Could you check a few things on this model? Use its own coordinates, in mm. A direction names the side the tool comes from. Give positions to 0.01 mm unless a question says otherwise; leave off trailing zeros. Loops run counter-clockwise (first coordinate to the right, second up) from the corner with the lowest first, then second, coordinate; pieces in that order, holes last.
1. Imagine slicing it at A-A (y = 17.5). List the corners of the cut face in (x, z) for me, plus the area to 3 significant figures.
2. Thinking about a two-plate mould opening in Y: for faces 3 (the flat face through (31, -61.113, -3)), 4 (the flat face through (-1, -64.923, -3)), 5 (the flat face through (-68.834, -48, -3)), which applies, +Y half, -Y half, draft (parallel to the pull), parting line (faces both ways), or undercut?
3. For faces 1 (the flat face through (-66, -40, -3)), 2 (the flat face through (-48.11, -15.82, -2.63)), which set-ups out of +Z, -Z, +X, -X, +Y, -Y let a thin tool reach every point of the face, with its end or its side?
4. Imagine slicing it at C-C (x = -34). List the corners of the cut face in (y, z) for me, plus the area to 3 significant figures.
5. I need wall thicknesses on line 1 along X through (y, z) = (1, -2.8); line 2 along X through (y, z) = (-35, -1.9); line 3 along Y through (x, z) = (-37, -2.05). Which ranges of each line are inside material? Lowest first, please.
6. Imagine slicing it at B-B (x = 13). List the corners of the cut face in (y, z) for me, plus the area to 3 significant figures.
7. Imagine slicing it at D-D (z = -2.6). Count the separate pieces of the cut face and the enclosed holes in it, plus the area to 3 significant figures.
8. For P1, Ø1.6, axis at y = 32, z = -3, coming from the +X side; P2, Ø8, axis at x = -30.5, y = -17.5, coming from the -Z side; P3, Ø2.5, axis at y = 5, z = -4, coming from the -X side, each with a flat end and sliding along its axis, tell me the tip position at first contact or that it passes through.
```python
from build123d import *

# Parameters (mm, degrees)
SKETCH1_W                = 127
SKETCH1_H                = 80
TOP_DEPTH                = 5.334
SKETCH2_W                = 127
SKETCH2_H                = 5.334
BOTTOM_DEPTH             = 24.923365698
SKETCH4_W                = 5.334
SKETCH4_H                = 15.24
SKETCH4_H_2              = 12.7
RIGHTTOOTH_DEPTH         = 5.334
SKETCH5_W                = 5.334
SKETCH5_H                = 15.24
SKETCH5_H_2              = 12.7
LEFTTOOTH_DEPTH          = 5.334
SKETCH6_R                = 1.775
PERFBOARDSCREWCUTS_DEPTH = 95.771380308
DESIGN_DEPTH             = 5.334


with BuildPart() as part:
    # Sketch1 → Top (new body)
    with BuildSketch(Plane.XY):
        Rectangle(SKETCH1_W, SKETCH1_H)
    extrude(amount=-TOP_DEPTH)

    # Sketch2 → Bottom (add)
    with BuildSketch(Plane.XZ.offset(40)):
        with Locations((0, -2.667)):
            Rectangle(SKETCH2_W, SKETCH2_H)
    extrude(amount=BOTTOM_DEPTH)

    # Sketch4 → RightTooth (add)
    with BuildSketch(Plane(origin=(63.5, 0, 0), x_dir=(0, 0, -1), z_dir=(1, 0, 0))):
        with Locations((2.667, -47.62)):
            Rectangle(SKETCH4_W, SKETCH4_H)
        with Locations((2.667, 17.15)):
            Rectangle(SKETCH4_W, SKETCH4_H_2)
    extrude(amount=RIGHTTOOTH_DEPTH)

    # Sketch5 → LeftTooth (add)
    with BuildSketch(Plane.ZY.offset(63.5)):
        with Locations((-2.667, -47.62)):
            Rectangle(SKETCH5_W, SKETCH5_H)
        with Locations((-2.667, 17.15)):
            Rectangle(SKETCH5_W, SKETCH5_H_2)
    extrude(amount=LEFTTOOTH_DEPTH)

    # Sketch6 → PerfBoardScrewCuts (cut, through all)
    with BuildSketch(Plane.XY):
        with Locations((-50.546, 34.544)):
            Circle(SKETCH6_R)
        with Locations((50.546, 34.544)):
            Circle(SKETCH6_R)
        with Locations((50.546, -34.544)):
            Circle(SKETCH6_R)
        with Locations((-50.546, -34.544)):
            Circle(SKETCH6_R)
    extrude(amount=-PERFBOARDSCREWCUTS_DEPTH, mode=Mode.SUBTRACT)

    # Sketch7 → Design (cut)
    with BuildSketch(Plane.XY):
        Polygon((-36.205413156, -0.032550322), (-59.69, 31.11), (-59.69, -31.175100644), align=None)
        Polygon((-41.91, 24.76), (-45.9906408, 24.76), (-31.75, 5.87570471), (-8.89, 36.19), (-41.91, 36.19), align=None)
        Polygon((-8.89, -36.255100644), (-31.75, -5.940805354), (-49.821467111, -29.905100644), (-41.91, -29.905100644), (-41.91, -36.255100644), align=None)
        Polygon((-3.81, 31.11), (-27.294586844, -0.032550322), (-3.81, -31.175100644), align=None)
        Polygon((3.81, -31.175100644), (27.294586844, -0.032550322), (3.81, 31.11), align=None)
        Polygon((45.9906408, 24.76), (41.91, 24.76), (41.91, 36.19), (8.89, 36.19), (31.75, 5.87570471), align=None)
        Polygon((59.69, 31.11), (36.205413156, -0.032550322), (59.69, -31.175100644), align=None)
        Polygon((49.821467111, -29.905100644), (31.75, -5.940805354), (8.89, -36.255100644), (41.91, -36.255100644), (41.91, -29.905100644), align=None)
        Polygon((55.88, -43.875100644), (7.62, -43.875100644), (31.75, -50.097955181), align=None)
        Polygon((59.69, -47.685100644), (41.041907363, -52.494233171), (59.69, -57.303365698), align=None)
        Polygon((55.88, -61.113365698), (31.75, -54.890511161), (7.62, -61.113365698), align=None)
        Polygon((3.81, -57.303365698), (22.458092637, -52.494233171), (3.81, -47.685100644), align=None)
        Polygon((-3.81, -47.685100644), (-22.458092637, -52.494233171), (-3.81, -57.303365698), align=None)
        Polygon((-55.88, -43.875100644), (-31.75, -50.097955181), (-7.62, -43.875100644), align=None)
        Polygon((-41.041907363, -52.494233171), (-59.69, -47.685100644), (-59.69, -57.303365698), align=None)
        Polygon((-7.62, -61.113365698), (-31.75, -54.890511161), (-55.88, -61.113365698), align=None)
    extrude(amount=-DESIGN_DEPTH, mode=Mode.SUBTRACT)


solid = part.part
```
Derived:
1. outline: (-68.83, -5.33) - (-59.69, -5.33) - (-59.69, 0) - (-68.83, 0) - close; (-49.43, -5.33) - (-40.52, -5.33) - (-40.52, 0) - (-49.43, 0) - close; (-22.98, -5.33) - (-14.07, -5.33) - (-14.07, 0) - (-22.98, 0) - close; (-3.81, -5.33) - (3.81, -5.33) - (3.81, 0) - (-3.81, 0) - close; (14.07, -5.33) - (22.98, -5.33) - (22.98, 0) - (14.07, 0) - close; (40.52, -5.33) - (49.43, -5.33) - (49.43, 0) - (40.52, 0) - close; (59.69, -5.33) - (68.83, -5.33) - (68.83, 0) - (59.69, 0) - close
1. area: 328 mm2
2. face 3: undercut
2. face 4: -Y half
2. face 5: draft
3. face 1: +Z, -Z, -X
3. face 2: +Z, -Z
4. outline: (-64.92, -5.33) - (-61.11, -5.33) - (-61.11, 0) - (-64.92, 0) - close; (-55.47, -5.33) - (-49.52, -5.33) - (-49.52, 0) - (-55.47, 0) - close; (-43.88, -5.33) - (-36.26, -5.33) - (-36.26, 0) - (-43.88, 0) - close; (-8.92, -5.33) - (8.86, -5.33) - (8.86, 0) - (-8.92, 0) - close; (36.19, -5.33) - (40, -5.33) - (40, 0) - (36.19, 0) - close
4. area: 208 mm2
5. line 1: x = -63.5 to -59.69, -36.98 to -26.52, -3.81 to 3.81, 26.52 to 36.98, 59.69 to 63.5
5. line 2: x = -63.5 to -52.26, -48.83 to -41.91, -9.84 to 9.84, 41.91 to 48.83, 52.26 to 63.5
5. line 3: y = -64.92 to -61.11, -56.24 to -48.74, -43.88 to -36.26, -12.9 to -1.09, 1.02 to 12.84, 36.19 to 40
6. outline: (-64.92, -5.33) - (-61.11, -5.33) - (-61.11, 0) - (-64.92, 0) - close; (-59.73, -5.33) - (-54.93, -5.33) - (-54.93, 0) - (-59.73, 0) - close; (-50.06, -5.33) - (-45.26, -5.33) - (-45.26, 0) - (-50.06, 0) - close; (-43.88, -5.33) - (-36.26, -5.33) - (-36.26, 0) - (-43.88, 0) - close; (-30.8, -5.33) - (-18.99, -5.33) - (-18.99, 0) - (-30.8, 0) - close; (18.92, -5.33) - (30.74, -5.33) - (30.74, 0) - (18.92, 0) - close; (36.19, -5.33) - (40, -5.33) - (40, 0) - (36.19, 0) - close
6. area: 258 mm2
7. separate pieces: 1
7. enclosed holes: 20
7. area: 7,250 mm2
8. P1: stops at x = 63.5
8. P2: passes through
8. P3: stops at x = -63.5
